from build123d import *

# Parameters (mm, degrees)
F1_DEPTH = 3


with BuildPart() as f1:
    # F0 (on Front) → F1 (new body)
    with BuildSketch(Plane.XZ):
        Polygon((13, 0), (10, 1.5838444032), (10, -1.5838444032), align=None)
        Polygon((10, -1.5838444032), (10, 1.5838444032), (9.0211303259, 4.5964954843), (7.1592095616, 7.1592095616), (4.5964954843, 9.0211303259), (1.5838444032, 10), (-1.5838444032, 10), (-4.5964954843, 9.0211303259), (-7.1592095616, 7.1592095616), (-9.0211303259, 4.5964954843), (-10, 1.5838444032), (-10, -1.5838444032), (-9.0211303259, -4.5964954843), (-7.1592095616, -7.1592095616), (-4.5964954843, -9.0211303259), (-1.5838444032, -10), (1.5838444032, -10), (4.5964954843, -9.0211303259), (7.1592095616, -7.1592095616), (9.0211303259, -4.5964954843), align=None)
        Polygon((9.0211303259, 4.5964954843), (10, 1.5838444032), (12.3637347118, 4.0172209269), align=None)
        Polygon((12.3637347118, -4.0172209269), (10, -1.5838444032), (9.0211303259, -4.5964954843), align=None)
        Polygon((7.1592095616, 7.1592095616), (9.0211303259, 4.5964954843), (10.5172209269, 7.6412082798), align=None)
        Polygon((10.5172209269, -7.6412082798), (9.0211303259, -4.5964954843), (7.1592095616, -7.1592095616), align=None)
        Polygon((4.5964954843, 9.0211303259), (7.1592095616, 7.1592095616), (7.6412082798, 10.5172209269), align=None)
        Polygon((7.6412082798, -10.5172209269), (7.1592095616, -7.1592095616), (4.5964954843, -9.0211303259), align=None)
        Polygon((1.5838444032, 10), (4.5964954843, 9.0211303259), (4.0172209269, 12.3637347118), align=None)
        Polygon((4.0172209269, -12.3637347118), (4.5964954843, -9.0211303259), (1.5838444032, -10), align=None)
        Polygon((-1.5838444032, 10), (1.5838444032, 10), (0, 13), align=None)
        Polygon((0, -13), (1.5838444032, -10), (-1.5838444032, -10), align=None)
        Polygon((-4.5964954843, 9.0211303259), (-1.5838444032, 10), (-4.0172209269, 12.3637347118), align=None)
        Polygon((-4.0172209269, -12.3637347118), (-1.5838444032, -10), (-4.5964954843, -9.0211303259), align=None)
        Polygon((-7.1592095616, 7.1592095616), (-4.5964954843, 9.0211303259), (-7.6412082798, 10.5172209269), align=None)
        Polygon((-7.6412082798, -10.5172209269), (-4.5964954843, -9.0211303259), (-7.1592095616, -7.1592095616), align=None)
        Polygon((-9.0211303259, 4.5964954843), (-7.1592095616, 7.1592095616), (-10.5172209269, 7.6412082798), align=None)
        Polygon((-10.5172209269, -7.6412082798), (-7.1592095616, -7.1592095616), (-9.0211303259, -4.5964954843), align=None)
        Polygon((-10, 1.5838444032), (-9.0211303259, 4.5964954843), (-12.3637347118, 4.0172209269), align=None)
        Polygon((-12.3637347118, -4.0172209269), (-9.0211303259, -4.5964954843), (-10, -1.5838444032), align=None)
        Polygon((-10, -1.5838444032), (-10, 1.5838444032), (-13, 0), align=None)
    extrude(amount=F1_DEPTH)


solid = f1.part
Input: part model. Units: mm. Frame: model coordinates. A direction names the side the tool comes from. Give positions to 0.01 mm unless a question says otherwise; leave off trailing zeros. Write each loop counter-clockwise with the first axis right and the second up, starting at its lowest first coordinate (ties: lowest second). Pieces come first, ordered by that corner, then holes.
Q1. Set-up query: faces 1 (the face through (-9.76, -1.48, -6.1)), 2 (the face through (10.67, -1.48, -4.31)), 3 (the face through (6.1, -1.48, -9.76)). Return all of +Z, -Z, +X, -X, +Y, -Y with unobstructed straight access to the full face (end or side cutting, diameter ignored); none if empty.
Q2. Pull-direction query (X, two-part tool) for faces 4 (the face through (-10.67, -1.48, 4.31)), 5 (the face through (2.82, -1.48, 11.2)), 6 (the face through (11.479, -1.479, -0.803)); classes: pulls with the +X half, pulls with the -X half, needs draft (parallel to the pull), parting line crosses it, or undercut.
Q3. First-contact query: P1, Ø1.5, axis at y = -1, z = -3.5, coming from the -X side. Flat tip, straight axial feed; report the tip coordinate or a pass-through.
Q4. Material intervals for probe 1 along X at (y, z) = (-2, 10.25); probe 2 along Z at (x, y) = (-10.75, -1.6); probe 3 along Z at (x, y) = (9.75, -0.5), sorted ascending.
Q5. Section A-A, the plane x = -8.5. Output: boundary loops of the cut face in (y, z), plus the area to 3 significant figures.
Q6. Section B-B, the plane z = -5.75. Output: boundary loops of the cut face in (x, y).
Filled in:
1. face 1: -X, +Y, -Y
1. face 2: +X, +Y, -Y
1. face 3: -Z, +Y, -Y
2. face 4: pulls with the -X half
2. face 5: undercut
2. face 6: pulls with the +X half
3. P1: stops at x = -12.36
4. probe 1: x = -7.6 to -7.1, -4.38 to -1.84, -1.45 to 1.45, 1.84 to 4.38, 7.1 to 7.6
4. probe 2: z = -4.3 to -2.36, -1.19 to 1.19, 2.36 to 4.3
4. probe 3: z = -7.53 to -6.08, -4.47 to 4.47, 6.08 to 7.53
5. outline: (-3, -7.35) - (0, -7.35) - (0, 7.35) - (-3, 7.35) - close
5. area: 44.1 mm2
6. outline: (-9.59, -3) - (9.59, -3) - (9.59, 0) - (-9.59, 0) - close
